Can you work these out from the model? Positions are in its coordinate system, mm. Face numbers are marked on the shaded views. Round coordinates to 2 decimals unless told otherwise and drop trailing zeros. Loops run counter-clockwise (first coordinate to the right, second up) from the corner with the lowest first, then second, coordinate; pieces in that order, holes last.
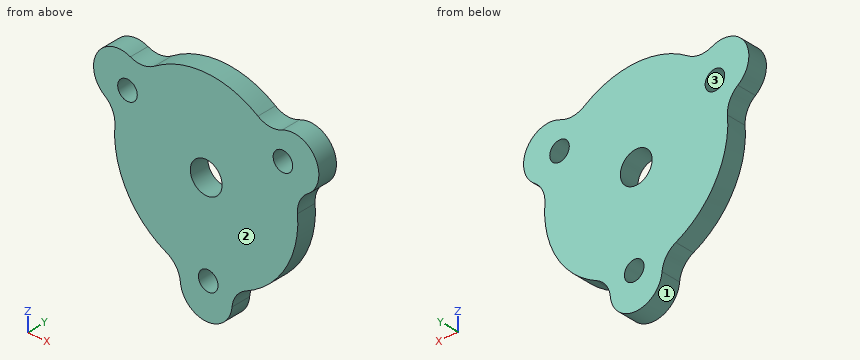
from build123d import *

# Parameters (mm, degrees)
SKETCH1_R           = 2.6
BOSS_EXTRUDE1_DEPTH = 3.175
FILLET1_R           = 4
SKETCH2_R           = 1.6
CUT_EXTRUDE1_DEPTH  = 4.1750001


with BuildPart() as part:
    # Sketch1 → Boss-Extrude1 (new body)
    with BuildSketch(Plane(origin=(0, 0, 0), x_dir=(1, 0, 0), z_dir=(0, 1, 0))):
        with BuildLine():
            Line((-4.25, 16.385322381), (-4.25, 14.385322381))
            ThreePointArc((-4.25, 14.385322381), (-12.990381057, 7.5), (-14.583054623, -3.512053224))
            Line((-14.583054623, -3.512053224), (-16.315105431, -4.512053224))
            ThreePointArc((-16.315105431, -4.512053224), (-17.870713397, -10.31766119), (-12.065105431, -11.873269156))
            Line((-12.065105431, -11.873269156), (-10.333054623, -10.873269156))
            ThreePointArc((-10.333054623, -10.873269156), (0, -15), (10.333054623, -10.873269156))
            Line((10.333054623, -10.873269156), (12.065105431, -11.873269156))
            ThreePointArc((12.065105431, -11.873269156), (17.870713397, -10.31766119), (16.315105431, -4.512053224))
            Line((16.315105431, -4.512053224), (14.583054623, -3.512053224))
            ThreePointArc((14.583054623, -3.512053224), (12.990381057, 7.5), (4.25, 14.385322381))
            Line((4.25, 14.385322381), (4.25, 16.385322381))
            ThreePointArc((4.25, 16.385322381), (0, 20.635322381), (-4.25, 16.385322381))
        make_face()
        Circle(SKETCH1_R, mode=Mode.SUBTRACT)
    extrude(amount=BOSS_EXTRUDE1_DEPTH)

    # Fillet1
    fillet1_edges = [part.edges().sort_by_distance(p)[0] for p in [
        (-14.583054623, 1.5875, 3.512053224),
        (-4.25, 1.5875, -14.385322381),
        (4.25, 1.5875, -14.385322381),
        (14.583054623, 1.5875, 3.512053224),
        (10.333054623, 1.5875, 10.873269156),
        (-10.333054623, 1.5875, 10.873269156),
    ]]
    fillet(fillet1_edges, radius=FILLET1_R)

    # Sketch2 → Cut-Extrude1 (cut, through all)
    with BuildSketch(Plane(origin=(0, 3.175, 0), x_dir=(1, 0, 0), z_dir=(0, 1, 0))):
        with Locations((-12.88502754, -7.05928361)):
            Circle(SKETCH2_R)
        with Locations((12.556032709, -7.629119373)):
            Circle(SKETCH2_R)
        with Locations((0.328994831, 14.688402983)):
            Circle(SKETCH2_R)
    extrude(amount=-CUT_EXTRUDE1_DEPTH, mode=Mode.SUBTRACT)


solid = part.part
(1) If we section it at A-A, the plane z = 0: List the corners of the cut face in (x, y) for me (3 decimals).
Worked answers:
outline: (-15, 0) - (-2.6, 0) - (-2.6, 3.175) - (-15, 3.175) - close; (2.6, 0) - (15, 0) - (15, 3.175) - (2.6, 3.175) - close
(2) If we section it at B-B, the plane x = 0: List the corners of the cut face in (y, z) for me (3 decimals).
Worked answers:
outline: (0, -20.635) - (3.175, -20.635) - (3.175, -16.254) - (0, -16.254) - close; (0, -13.123) - (3.175, -13.123) - (3.175, -2.6) - (0, -2.6) - close; (0, 2.6) - (3.175, 2.6) - (3.175, 15) - (0, 15) - close
(3) If we mould it in two halves opening along Z, with no side actions, what happens to the marked faces 1, 2 and 3? For each: released by +Z, released by -Z, zero draft, split by the parting line, or undercut.
Worked answers:
face 1: released by -Z
face 2: zero draft
face 3: undercut
(4) If I drill on line 1 (X direction, y = 0.95, z = 0); line 2 (Z direction, x = 0, y = 2); line 3 (X direction, y = 2.5, z = -15), over which ranges is the centre line in solid material (lowest first)?
Worked answers:
line 1: x = -15 to -2.6, 2.6 to 15
line 2: z = -20.64 to -16.25, -13.12 to -2.6, 2.6 to 15
line 3: x = -4.83 to -1.24, 1.9 to 4.83
(5) If we section it at D-D, the plane y = 1.35: State how many separate pieces and enclosed holes the cut face has, then the cut area to 3 significant figures.
Worked answers:
separate pieces: 1
enclosed holes: 4
area: 794 mm2
(6) Will these pins go through, and if not, where does the flat tip stop? P1, Ø4, axis at x = -12, z = 6.5, coming from the -Y side; P2, Ø4, axis at x = 0, z = 0, coming from the +Y side.
Worked answers:
P1: stops at y = 0
P2: passes through
(7) If we section it at C-C, the plane z = -9: List the corners of the cut face in (x, y) for me (3 decimals), then the cut area to 3 significant figures.
Worked answers:
outline: (-12, 0) - (12, 0) - (12, 3.175) - (-12, 3.175) - close
area: 76.2 mm2
